from build123d import *

# Parameters (mm, degrees)
SKETCH1_R                                     = 76.2
BOSS_EXTRUDE1_DEPTH                           = 25.4
CBORE_FOR_3_8_BUTTON_HEAD_CAP_SCREW1_AT_COUNT = 2
CBORE_FOR_3_8_BUTTON_HEAD_CAP_SCREW1_AT_PITCH = 75.078270051
CBORE_FOR_3_8_BUTTON_HEAD_CAP_SCREW1_2_COUNT  = 2
CBORE_FOR_3_8_BUTTON_HEAD_CAP_SCREW1_2_PITCH  = 60.736241383
CBORE_FOR_3_8_BUTTON_HEAD_CAP_SCREW1_3_COUNT  = 2
CBORE_FOR_3_8_BUTTON_HEAD_CAP_SCREW1_3_PITCH  = 85.541398896
CBORE_FOR_3_8_BUTTON_HEAD_CAP_SCREW1_4_COUNT  = 2
CBORE_FOR_3_8_BUTTON_HEAD_CAP_SCREW1_4_PITCH  = 57.302034519


with BuildPart() as part:
    # Sketch1 → Boss-Extrude1 (new body)
    with BuildSketch(Plane(origin=(0, 0, 0), x_dir=(1, 0, 0), z_dir=(0, 1, 0))):
        with Locations(Location((0, 0, 0), (0, 0, 270))):
            Circle(SKETCH1_R)
    extrude(amount=-BOSS_EXTRUDE1_DEPTH)

    # Sketch4 → CBORE for 3/8 Button Head Cap Screw1 (revolve, cut)
    with BuildSketch(Plane(origin=(60.58130803, 0, -11.552884304), x_dir=(0, 0, 1), z_dir=(1, 0, 0))):
        Polygon((0, 0), (0, 25.4), (5.0419, 25.4), (5.0419, 5.0546), (8.73125, 5.0546), (8.73125, 0.635), (9.36625, 0), align=None)
    cbore_for_3_8_button_head_cap_screw1 = revolve(axis=Axis((60.58130803, 6.35, -11.552884304), (0, -1, 0)), mode=Mode.SUBTRACT)

    # CBORE for 3/8 Button Head Cap Screw1 at: CBORE for 3/8 Button Head Cap Screw1 ×2
    with Locations(*[Vector(-0.5918446125142773, 0, 0.8060520793582913) * (i * CBORE_FOR_3_8_BUTTON_HEAD_CAP_SCREW1_AT_PITCH) for i in range(1, CBORE_FOR_3_8_BUTTON_HEAD_CAP_SCREW1_AT_COUNT)]):
        add(cbore_for_3_8_button_head_cap_screw1, mode=Mode.SUBTRACT)

    # CBORE for 3_8 Button Head Cap Screw1 2: CBORE for 3/8 Button Head Cap Screw1 ×2
    with Locations(*[Vector(-0.8654863573421582, 0, 0.5009324957063599) * (i * CBORE_FOR_3_8_BUTTON_HEAD_CAP_SCREW1_2_PITCH) for i in range(1, CBORE_FOR_3_8_BUTTON_HEAD_CAP_SCREW1_2_COUNT)]):
        add(cbore_for_3_8_button_head_cap_screw1, mode=Mode.SUBTRACT)

    # CBORE for 3_8 Button Head Cap Screw1 3: CBORE for 3/8 Button Head Cap Screw1 ×2
    with Locations(*[Vector(-0.9738464853959384, 0, -0.22720700447384592) * (i * CBORE_FOR_3_8_BUTTON_HEAD_CAP_SCREW1_3_PITCH) for i in range(1, CBORE_FOR_3_8_BUTTON_HEAD_CAP_SCREW1_3_COUNT)]):
        add(cbore_for_3_8_button_head_cap_screw1, mode=Mode.SUBTRACT)

    # CBORE for 3_8 Button Head Cap Screw1 4: CBORE for 3/8 Button Head Cap Screw1 ×2
    with Locations(*[Vector(-0.7754466315152058, 0, -0.6314131149031676) * (i * CBORE_FOR_3_8_BUTTON_HEAD_CAP_SCREW1_4_PITCH) for i in range(1, CBORE_FOR_3_8_BUTTON_HEAD_CAP_SCREW1_4_COUNT)]):
        add(cbore_for_3_8_button_head_cap_screw1, mode=Mode.SUBTRACT)


solid = part.part
For this review, take the finished solid that the model builds, in its own axes (mm). A direction names the side the tool comes from. Round coordinates to 2 decimals unless told otherwise and drop trailing zeros. Order: outer loops, then holes, each group sorted by start corner. A loop starts at its lowest first (then second) coordinate and runs counter-clockwise, first axis right, second up. Notation, with made-up numbers: (73, 4.25) -> (89, 4.25) arc R27 ccw to (89, 33.25) -> close; hole circle Ø6 at (68.5, -21). An arc over 180 degrees is marked (long way). Put each result on its own line as item: value.
Q1. Add section C-C on z = 65. Write out the cut boundary in (x, y).
Check result:
outline: (-39.77, -25.4) -> (39.77, -25.4) -> (39.77, 0) -> (-39.77, 0) -> close
Q2. Machinability: for faces 1 (the flat face through (1, -25.4, -1)), 2 (the cylindrical face through (-23.11, -2.81, -39.71)), which of the approach directions +Z, -Z, +X, -X, +Y, -Y give a long, thin tool a straight path to every point of the face, cutting with its end or side? Answer none if there is none.
Check result:
face 1: +Z, -Z, +X, -X, -Y
face 2: +Y
Q3. For probe 1 along Z at (x, y) = (13.5, -23); probe 2 along Y at (x, z) = (57, -18.5); probe 3 along Z at (x, y) = (-25, -22.5), list the stretches that pass through material, from the lowest coordinate up. Write a range as [from, to].
Check result:
probe 1: [-74.99, -52.03], [-43.44, 44.67], [53.26, 74.99]
probe 2: [-25.4, -5.05]
probe 3: [-71.98, -35.49], [-26.49, 71.98]
Q4. Insertion check: pin 1 Ø10 at (x, z) = (-2, -36) entering from +Y; pin 2 Ø1 at (y, z) = (-12.5, 24.5) entering from +X; pin 3 Ø15.5 at (x, z) = (8.01, 18.87) entering from +Y; pin 4 Ø4 at (y, z) = (-20, 14) entering from +X. Each pin has a flat end and moves straight along its axis. Give the tip position at first contact, or say it passes through.
Check result:
pin 1: y = 0
pin 2: x = 72.32
pin 3: y = -5.05
pin 4: x = 75.25
Q5. Mouldability with a two-part tool opening along Z and no side actions: class faces 3 (the cylindrical face through (-46.367, -12.522, -60.47)), 4 (the cylindrical face through (14.632, -15.085, -42.925)), 5 (the flat face through (1, 0, -1)) as pulls with the +Z half, pulls with the -Z half, needs draft (parallel to the pull), parting line crosses it, or undercut.
Check result:
face 3: parting line crosses it
face 4: undercut
face 5: needs draft
Q6. Add section B-B on x = -43. Write out the cut boundary in (y, z), plus the area to 3 significant figures.
Check result:
outline: (-25.4, -62.91) -> (0, -62.91) -> (0, 62.91) -> (-25.4, 62.91) -> close
area: 3,200 mm2
Q7. Add section A-A on y = -19. Write out the cut boundary in (x, z).
Check result:
outline: circle Ø152.4 at (0, 0); hole circle Ø10.08 at (-22.72, -30.99); hole circle Ø10.08 at (8.01, 18.87); hole circle Ø10.08 at (16.15, -47.73); hole circle Ø10.08 at (16.15, 48.96); hole circle Ø10.08 at (60.58, -11.55)
